Geometry check sheet. Reference: the model listing, model coordinates, mm. A direction names the side the tool comes from. Round coordinates to 2 decimals unless told otherwise and drop trailing zeros. Loops run counter-clockwise (first coordinate to the right, second up) from the corner with the lowest first, then second, coordinate; pieces in that order, holes last. Notation, with made-up numbers: M -7.5,17.5 L 27.5,17.5 A26 ccw 27.5,56.5 Z; hole C 32,75.25 d4. An arc over 180 degrees is marked long. Write item = value, one per line.
from build123d import *

# Parameters (mm, degrees)
SKETCH2_R           = 8
BOSS_EXTRUDE1_DEPTH = 25
SKETCH3_R           = 4.5
CUT_EXTRUDE1_DEPTH  = 15.13
SKETCH4_R           = 2.5
CUT_EXTRUDE2_DEPTH  = 10.87
FILLET1_R           = 0.5
FILLET2_R           = 0.5
CHAMFER1_SIZE       = 0.5
FILLET3_R           = 0.2


with BuildPart() as part:
    # Sketch2 → Boss-Extrude1 (new body)
    with BuildSketch(Plane(origin=(0, 0, 0), x_dir=(1, 0, 0), z_dir=(0, 1, 0))):
        Circle(SKETCH2_R)
    extrude(amount=BOSS_EXTRUDE1_DEPTH)

    # Sketch3 → Cut-Extrude1 (cut)
    with BuildSketch(Plane(origin=(0, 25, 0), x_dir=(1, 0, 0), z_dir=(0, 1, 0))):
        Circle(SKETCH3_R)
    extrude(amount=-CUT_EXTRUDE1_DEPTH, mode=Mode.SUBTRACT)

    # Sketch4 → Cut-Extrude2 (cut, through all)
    with BuildSketch(Plane(origin=(0, 9.87, 0), x_dir=(1, 0, 0), z_dir=(0, 1, 0))):
        Circle(SKETCH4_R)
    extrude(amount=-CUT_EXTRUDE2_DEPTH, mode=Mode.SUBTRACT)

    # Fillet1
    fillet1_edges = [part.edges().sort_by_distance(p)[0] for p in [
        (-8, 25, 0),
    ]]
    fillet(fillet1_edges, radius=FILLET1_R)

    # Fillet2
    fillet2_edges = [part.edges().sort_by_distance(p)[0] for p in [
        (-4.5, 25, 0),
    ]]
    fillet(fillet2_edges, radius=FILLET2_R)

    # Chamfer1
    chamfer1_edges = [part.edges().sort_by_distance(p)[0] for p in [
        (-2.5, 0, 0),
        (-2.5, 9.87, 0),
    ]]
    chamfer(chamfer1_edges, length=CHAMFER1_SIZE)

    # Fillet3
    fillet3_edges = [part.edges().sort_by_distance(p)[0] for p in [
        (-8, 0, 0),
    ]]
    fillet(fillet3_edges, radius=FILLET3_R)


solid = part.part
(1) Sectioned sample at C-C on y = 7.25. Record the cut outline in (x, z).
Result set:
outline = C 0,0 d16; hole C 0,0 d5
(2) Tool access check on faces 1 (the flat face through (1, 9.87, 3)), 2 (the flat face through (3.4, 0, -0.1)). Record the directions out of +Z, -Z, +X, -X, +Y, -Y that give a thin tool (end or side, any length) a straight path to the whole face; none if there is none.
Result set:
face_1 = +Y
face_2 = +Z, -Z, +X, -X, -Y
(3) Sectioned sample at D-D on y = 11.75. Record the cut outline in (x, z), then the cut area to 3 significant figures.
Result set:
outline = C 0,0 d16; hole C 0,0 d9
area = 137 mm2
(4) Release check for a two-part mould opening along X. For faces 3 (the flat face through (5, 25, 2)), 4 (the cylindrical face through (-1.73, 12.18, 7.81)), 5 (the cylindrical face through (-0.54, 5, 2.44)) record: released by +X, released by -X, zero draft, split by the parting line, or undercut.
Result set:
face_3 = zero draft
face_4 = split by the parting line
face_5 = undercut
(5) Sectioned sample at A-A on z = 0. Record the cut outline in (x, y).
Result set:
outline = M -8,0.2 A0.2 ccw -7.8,0 L -3,0 L -2.5,0.5 L -2.5,9.37 L -3,9.87 L -4.5,9.87 L -4.5,24.5 A0.5 ccw -5,25 L -7.5,25 A0.5 ccw -8,24.5 Z; M 2.5,0.5 L 3,0 L 7.8,0 A0.2 ccw 8,0.2 L 8,24.5 A0.5 ccw 7.5,25 L 5,25 A0.5 ccw 4.5,24.5 L 4.5,9.87 L 3,9.87 L 2.5,9.37 Z
(6) Material ranges on line 1 along Z through (x, y) = (0, 2.75); line 2 along X through (y, z) = (15.5, 0), recorded low to high. Write a range as from..to.
Result set:
line_1 = -8..-2.5, 2.5..8
line_2 = -8..-4.5, 4.5..8
(7) Sectioned sample at B-B on x = 0. Record the cut outline in (y, z), then the cut area to 3 significant figures.
Result set:
outline = M 0,-7.8 A0.2 ccw 0.2,-8 L 24.5,-8 A0.5 ccw 25,-7.5 L 25,-5 A0.5 ccw 24.5,-4.5 L 9.87,-4.5 L 9.87,-3 L 9.37,-2.5 L 0.5,-2.5 L 0,-3 Z; M 0,3 L 0.5,2.5 L 9.37,2.5 L 9.87,3 L 9.87,4.5 L 24.5,4.5 A0.5 ccw 25,5 L 25,7.5 A0.5 ccw 24.5,8 L 0.2,8 A0.2 ccw 0,7.8 Z
area = 214 mm2
(8) Depth check by flat-ended pin: pin 1 Ø8 at (x, z) = (0, 0) entering from +Y; pin 2 Ø8 at (x, y) = (-4.5, 5) entering from -Z; pin 3 Ø5.5 at (x, z) = (0, 0) entering from -Y. Enter the tip coordinate at first touch or a pass-through.
Result set:
pin_1 = 9.87
pin_2 = -7.98
pin_3 = 0.25
